from build123d import *

# Parameters (mm, degrees)
SKETCH_1_W      = 33
SKETCH_1_H      = 35
SKETCH_1_W_2    = 5
SKETCH_1_H_2    = 40
SKETCH_1_H_3    = 15.5
EXTRUDE_1_DEPTH = 5


with BuildPart() as part:
    # 草圖1 → 填料-伸長1 (new body)
    # profile 1 of 3: a face of its own
    with BuildSketch(Plane(origin=(0, 0, 0), x_dir=(1, 0, 0), z_dir=(0, 1, 0))):
        with BuildLine():
            Line((16.5, -27.5), (-16.5, -27.5))
            ThreePointArc((-16.5, -27.5), (-23.571067812, -24.571067812), (-26.5, -17.5))
            Line((-26.5, -17.5), (-26.5, 17.5))
            ThreePointArc((-26.5, 17.5), (-23.571067812, 24.571067812), (-16.5, 27.5))
            Line((-16.5, 27.5), (16.5, 27.5))
            ThreePointArc((16.5, 27.5), (23.571067812, 24.571067812), (26.5, 17.5))
            Line((26.5, 17.5), (26.5, -17.5))
            ThreePointArc((26.5, -17.5), (23.571067812, -24.571067812), (16.5, -27.5))
        make_face()
        Rectangle(SKETCH_1_W, SKETCH_1_H, mode=Mode.SUBTRACT)
    # profile 2 of 3: a face of its own
    with BuildSketch(Plane(origin=(0, 0, 0), x_dir=(1, 0, 0), z_dir=(0, 1, 0))):
        with Locations((18.607544966, -44.554985824)):
            Rectangle(SKETCH_1_W_2, SKETCH_1_H_2)
    # profile 3 of 3: a face of its own
    with BuildSketch(Plane(origin=(0, 0, 0), x_dir=(1, 0, 0), z_dir=(0, 1, 0))):
        with Locations((-4.392455034, -35.25)):
            Rectangle(SKETCH_1_W_2, SKETCH_1_H_3)
    extrude(amount=EXTRUDE_1_DEPTH)


solid = part.part
Work out the finished part from the listing and answer in its coordinate system (mm). A direction names the side the tool comes from. Round coordinates to 2 decimals unless told otherwise and drop trailing zeros. Loops run counter-clockwise (first coordinate to the right, second up) from the corner with the lowest first, then second, coordinate; pieces in that order, holes last. Notation, with made-up numbers: (35.5, 63.5) - (82.5, 63.5) arc R15 ccw to (82.5, 74.5) - close; hole circle Ø4 at (-19.75, 62.5). An arc over 180 degrees is marked (long way). Use one line per item in the form item = value. Start each with the question number.
(1) A flat-ended cylindrical pin translates along its axis: P1, Ø1.5, axis at x = 8.5, y = 2, coming from the +Z side. Find the tip coordinate at first contact, or state that the pin passes through.
(2) Which of the six approach directions +Z, -Z, +X, -X, +Y, -Y give full straight-line access (tool end or side, diameter ignored) to faces 4 (the face through (-6.892, 2, 35)), 5 (the face through (16.108, 2, 46)), 6 (the face through (21.108, 2, 46))?
(3) Find section B-B on y = 2.6. Determine the outline of the cut face in (x, z).
(4) Find section A-A on z = 33.5. Determine the outline of the cut face in (x, y), and give its area (3 significant figures).
(5) Consider line 1 (X direction, y = 3.8, z = -13); line 2 (Z direction, x = -4, y = 1.05); line 3 (Z direction, x = 9, y = 0.75). Determine where each line is inside the solid, lowest interval first.
(6) Find section D-D on z = 45. Determine the outline of the cut face in (x, y).
(7) Determine the mould class of faces 1 (the face through (23.49, 2.46, -24.65)), 2 (the face through (-16.5, 2, 0)), 3 (the face through (-26.5, 2, 0)) for opening direction Z: +Z half, -Z half, draft (parallel to the pull), parting line (faces both ways), or undercut.
(8) Find section C-C on x = 9. Determine the outline of the cut face in (y, z), and give its area (3 significant figures).
Answer list:
q1.P1 = 27.5
q2.face_4 = +Z, -X, +Y, -Y
q2.face_5 = +Z, +Y, -Y
q2.face_6 = +Z, +X, +Y, -Y
q3.outline = (-26.5, -17.5) arc R10 ccw to (-16.5, -27.5) - (16.5, -27.5) arc R10 ccw to (26.5, -17.5) - (26.5, 17.5) arc R10 ccw to (21.11, 26.38) - (21.11, 64.55) - (16.11, 64.55) - (16.11, 27.5) - (-1.89, 27.5) - (-1.89, 43) - (-6.89, 43) - (-6.89, 27.5) - (-16.5, 27.5) arc R10 ccw to (-26.5, 17.5) - close; hole (-16.5, -17.5) - (16.5, -17.5) - (16.5, 17.5) - (-16.5, 17.5) - close
q4.outline = (-6.89, 0) - (-1.89, 0) - (-1.89, 5) - (-6.89, 5) - close; (16.11, 0) - (21.11, 0) - (21.11, 5) - (16.11, 5) - close
q4.area = 50.0 mm^2
q5.line_1 = -26.5 to -16.5, 16.5 to 26.5
q5.line_2 = -27.5 to -17.5, 17.5 to 43
q5.line_3 = -27.5 to -17.5, 17.5 to 27.5
q6.outline = (16.11, 0) - (21.11, 0) - (21.11, 5) - (16.11, 5) - close
q7.face_1 = -Z half
q7.face_2 = undercut
q7.face_3 = draft
q8.outline = (0, -27.5) - (5, -27.5) - (5, -17.5) - (0, -17.5) - close; (0, 17.5) - (5, 17.5) - (5, 27.5) - (0, 27.5) - close
q8.area = 100 mm^2
